from build123d import *

# Parameters (mm, degrees)
SKETCH1_R           = 75
BOSS_EXTRUDE1_DEPTH = 70
CUT_EXTRUDE1_DEPTH  = 65
SKETCH3_3_W         = 1.992128126
SKETCH3_3_H         = 23
SKETCH3_3_W_2       = 2.893011501
CUT_EXTRUDE3_DEPTH  = 60
BOSS_EXTRUDE2_DEPTH = 65


with BuildPart() as part:
    # Sketch1 → Boss-Extrude1 (new body)
    with BuildSketch(Plane(origin=(0, 0, 0), x_dir=(1, 0, 0), z_dir=(0, 1, 0))):
        with Locations((-19.143760263, 2.851198337)):
            Circle(SKETCH1_R)
    extrude(amount=BOSS_EXTRUDE1_DEPTH)

    # Sketch3 → Cut-Extrude1 (cut)
    with BuildSketch(Plane(origin=(0, 70, 0), x_dir=(1, 0, 0), z_dir=(0, 1, 0))):
        with BuildLine():
            Line((34.969329, 14.351198337), (44.830844074, 14.351198337))
            ThreePointArc((44.830844074, 14.351198337), (-19.143760263, 67.851198337), (-83.118364599, 14.351198337))
            Line((-83.118364599, 14.351198337), (-73.256849525, 14.351198337))
            Line((-73.256849525, 14.351198337), (-73.256849525, -8.648801663))
            Line((-73.256849525, -8.648801663), (-83.118364599, -8.648801663))
            ThreePointArc((-83.118364599, -8.648801663), (-19.143760263, -62.148801663), (44.830844074, -8.648801663))
            Line((44.830844074, -8.648801663), (34.969329, -8.648801663))
            Line((34.969329, -8.648801663), (34.969329, 14.351198337))
        make_face()
    extrude(amount=-CUT_EXTRUDE1_DEPTH, mode=Mode.SUBTRACT)

    # Sketch3_3 → Cut-Extrude3 (cut)
    with BuildSketch(Plane(origin=(0, 70, 0), x_dir=(1, 0, 0), z_dir=(0, 1, 0))):
        with Locations((55.965393063, 2.851198337)):
            Rectangle(SKETCH3_3_W, SKETCH3_3_H)
        with BuildLine():
            Line((54.969329, -8.648801663), (54.969329, 14.351198337))
            Line((54.969329, 14.351198337), (44.830844074, 14.351198337))
            ThreePointArc((44.830844074, 14.351198337), (45.59938332, 8.624010396), (45.856239737, 2.851198337))
            ThreePointArc((45.856239737, 2.851198337), (45.59938332, -2.921613722), (44.830844074, -8.648801663))
            Line((44.830844074, -8.648801663), (54.969329, -8.648801663))
        make_face()
        with BuildLine():
            ThreePointArc((45.856239737, 2.851198337), (45.59938332, 8.624010396), (44.830844074, 14.351198337))
            Line((44.830844074, 14.351198337), (34.969329, 14.351198337))
            Line((34.969329, 14.351198337), (34.969329, -8.648801663))
            Line((34.969329, -8.648801663), (44.830844074, -8.648801663))
            ThreePointArc((44.830844074, -8.648801663), (45.59938332, -2.921613722), (45.856239737, 2.851198337))
        make_face()
        with BuildLine():
            Line((34.969329, 14.351198337), (44.830844074, 14.351198337))
            ThreePointArc((44.830844074, 14.351198337), (-19.143760263, 67.851198337), (-83.118364599, 14.351198337))
            Line((-83.118364599, 14.351198337), (-73.256849525, 14.351198337))
            Line((-73.256849525, 14.351198337), (-73.256849525, -8.648801663))
            Line((-73.256849525, -8.648801663), (-83.118364599, -8.648801663))
            ThreePointArc((-83.118364599, -8.648801663), (-19.143760263, -62.148801663), (44.830844074, -8.648801663))
            Line((44.830844074, -8.648801663), (34.969329, -8.648801663))
            Line((34.969329, -8.648801663), (34.969329, 14.351198337))
        make_face()
        with BuildLine():
            ThreePointArc((-83.118364599, -8.648801663), (-84.143760263, 2.851198337), (-83.118364599, 14.351198337))
            Line((-83.118364599, 14.351198337), (-93.256849525, 14.351198337))
            Line((-93.256849525, 14.351198337), (-93.256849525, -8.648801663))
            Line((-93.256849525, -8.648801663), (-83.118364599, -8.648801663))
        make_face()
        with BuildLine():
            Line((-73.256849525, 14.351198337), (-83.118364599, 14.351198337))
            ThreePointArc((-83.118364599, 14.351198337), (-84.143760263, 2.851198337), (-83.118364599, -8.648801663))
            Line((-83.118364599, -8.648801663), (-73.256849525, -8.648801663))
            Line((-73.256849525, -8.648801663), (-73.256849525, 14.351198337))
        make_face()
        with Locations((-94.703355276, 2.851198337)):
            Rectangle(SKETCH3_3_W_2, SKETCH3_3_H)
    extrude(amount=-CUT_EXTRUDE3_DEPTH, mode=Mode.SUBTRACT)

    # Sketch6 → Boss-Extrude2 (add)
    with BuildSketch(Plane(origin=(0, 5, 0), x_dir=(1, 0, 0), z_dir=(0, 1, 0))):
        with BuildLine():
            ThreePointArc((-80.485018809, 24.351198337), (-82.000871018, 19.403649138), (-83.118364599, 14.351198337))
            Line((-83.118364599, 14.351198337), (-73.256849525, 14.351198337))
            Line((-73.256849525, 14.351198337), (-73.256849525, 24.351198337))
            Line((-73.256849525, 24.351198337), (-80.485018809, 24.351198337))
        make_face()
        Polygon((-63.256849525, 24.351198337), (-63.256849525, -18.648801663), (-73.256849525, -18.648801663), (-73.256849525, -8.648801663), (-73.256849525, 14.351198337), (-73.256849525, 24.351198337), align=None)
        with BuildLine():
            Line((-73.256849525, -18.648801663), (-73.256849525, -8.648801663))
            Line((-73.256849525, -8.648801663), (-83.118364599, -8.648801663))
            ThreePointArc((-83.118364599, -8.648801663), (-82.000871018, -13.701252464), (-80.485018809, -18.648801663))
            Line((-80.485018809, -18.648801663), (-73.256849525, -18.648801663))
        make_face()
        Polygon((34.969329, 24.351198337), (24.969329, 24.351198337), (24.969329, -18.648801663), (34.969329, -18.648801663), (34.969329, -8.648801663), (34.969329, 14.351198337), align=None)
        with BuildLine():
            Line((34.969329, -18.648801663), (42.197498283, -18.648801663))
            ThreePointArc((42.197498283, -18.648801663), (43.713350492, -13.701252464), (44.830844074, -8.648801663))
            Line((44.830844074, -8.648801663), (34.969329, -8.648801663))
            Line((34.969329, -8.648801663), (34.969329, -18.648801663))
        make_face()
        with BuildLine():
            ThreePointArc((44.830844074, 14.351198337), (43.713350492, 19.403649138), (42.197498283, 24.351198337))
            Line((42.197498283, 24.351198337), (34.969329, 24.351198337))
            Line((34.969329, 24.351198337), (34.969329, 14.351198337))
            Line((34.969329, 14.351198337), (44.830844074, 14.351198337))
        make_face()
    extrude(amount=BOSS_EXTRUDE2_DEPTH)


solid = part.part
Can you work these out from the model? Positions are in its coordinate system, mm. A direction names the side the tool comes from. Coordinates: 2 decimals unless noted, no trailing zeros. Write each loop counter-clockwise with the first axis right and the second up, starting at its lowest first coordinate (ties: lowest second). Pieces come first, ordered by that corner, then holes. Notation, with made-up numbers: (39, 76.25) -> (56, 76.25) arc R23 cw to (56, 107.25) -> close; hole circle Ø3 at (2.5, 76.5). An arc over 180 degrees is marked (long way). Write each question's results on one line, items separated by ' | '. Start each with the question number.
Item 1: Thinking about a two-plate mould opening in Z: for faces 1 (the flat face through (-83, 40, -14.351)), 2 (the flat face through (-20, 0, -4)), 3 (the cylindrical face through (52.393, 34.51, -25.379)), which applies, released by +Z, released by -Z, zero draft, split by the parting line, or undercut?
Item 2: If we section it at C-C, the plane x = 19: Write out the boundary of the cut face in (y, z), and give its area (3 significant figures).
Item 3: On a 3-axis mill with a long thin cutter (end or side, diameter ignored), from which of +Z, -Z, +X, -X, +Y, -Y can I reach the whole of each face in a straight line? I mean faces 4 (the flat face through (45, 10, -3)), 5 (the flat face through (-73.257, 40, -3)), 6 (the flat face through (-72, 37, 18.649)). Say none if no direction works.
Item 4: I'm going to push flat-ended pins straight in: P1, Ø19, axis at x = -70, y = 47, coming from the +Z side; P2, Ø18.5, axis at y = 33.5, z = -5, coming from the -X side; P3, Ø13, axis at y = 35.5, z = -10.5, coming from the +X side. Where does each tip first touch, or does it pass through?
Item 5: If we section it at D-D, the plane x = -71: Write out the boundary of the cut face in (y, z), and give its area (3 significant figures).
Item 6: Please list where these lines run through material, in increasing order: probe 1 along X at (y, z) = (47.5, -4.5); probe 2 along Z at (x, y) = (-67, 46); probe 3 along Z at (x, y) = (-71, 20.5).
Item 7: If we section it at A-A, the plane y = 12.5: Write out the boundary of the cut face in (x, z), and give its area (3 significant figures).
Item 8: If we section it at B-B, the plane z = 27: Write out the boundary of the cut face in (x, y), and give its area (3 significant figures).
Answer block:
1) face 1: undercut | face 2: zero draft | face 3: split by the parting line
2) outline: (0, -67.43) -> (70, -67.43) -> (70, -55.48) -> (5, -55.48) -> (5, 49.78) -> (70, 49.78) -> (70, 61.72) -> (0, 61.72) -> close | area: 2,200 mm²
3) face 4: +X, +Y | face 5: -X, +Y | face 6: +Y
4) P1: z = 59.72 | P2: x = -73.26 | P3: x = 54.97
5) outline: (0, -57.04) -> (70, -57.04) -> (70, -42.04) -> (5, -42.04) -> (5, -24.35) -> (70, -24.35) -> (70, 18.65) -> (5, 18.65) -> (5, 36.34) -> (70, 36.34) -> (70, 51.33) -> (0, 51.33) -> close | area: 5,290 mm²
6) probe 1: -73.26 to -63.26, 24.97 to 34.97 | probe 2: -60.6 to -46.84, -24.35 to 18.65, 41.13 to 54.9 | probe 3: -57.04 to -42.04, -24.35 to 18.65, 36.34 to 51.33
7) outline: (-93.26, -14.35) arc R75 ccw to (54.97, -14.35) -> (34.97, -14.35) -> (34.97, 8.65) -> (54.97, 8.65) arc R75 ccw to (-93.26, 8.65) -> (-73.26, 8.65) -> (-73.26, -14.35) -> close; hole (-80.49, -24.35) arc R65 ccw to (42.2, -24.35) -> (24.97, -24.35) -> (24.97, 18.65) -> (42.2, 18.65) arc R65 ccw to (-80.49, 18.65) -> (-63.26, 18.65) -> (-63.26, -24.35) -> close | area: 5,140 mm²
8) outline: (-87.95, 0) -> (49.66, 0) -> (49.66, 70) -> (38.6, 70) -> (38.6, 5) -> (-76.88, 5) -> (-76.88, 70) -> (-87.95, 70) -> close | area: 2,130 mm²
